```python
from build123d import *

# Parameters (mm, degrees)
SKETCH_1_W          = 150
SKETCH_1_H          = 25
EXTRUDE_2_DEPTH     = 10
SKETCH_5_R          = 5.05
CUT_EXTRUDE_4_DEPTH = 77.689308251
FILLET_1_R          = 12.5


with BuildPart() as part:
    # Эскиз1 → Бобышка-Вытянуть2 (new body)
    with BuildSketch(Plane(origin=(0, 0, 0), x_dir=(1, 0, 0), z_dir=(0, 1, 0))):
        Rectangle(SKETCH_1_W, SKETCH_1_H)
    extrude(amount=EXTRUDE_2_DEPTH)

    # Эскиз5 → Вырез-Вытянуть4 (cut, through all)
    with BuildSketch(Plane(origin=(0, 10, 0), x_dir=(1, 0, 0), z_dir=(0, 1, 0))):
        with Locations(Location((-60, 0, 0), (0, 0, 270))):
            Circle(SKETCH_5_R)
    cut_extrude_4 = extrude(amount=-CUT_EXTRUDE_4_DEPTH, mode=Mode.SUBTRACT)

    # Зеркальное отражение1: Вырез-Вытянуть4 across plane
    add(cut_extrude_4.mirror(Plane(origin=(0, 0, 0), x_dir=(0, 0, 1), z_dir=(1, 0, 0))), mode=Mode.SUBTRACT)

    # Скругление1
    fillet_1_edges = [part.edges().sort_by_distance(p)[0] for p in [
        (-75, 5, 12.5),
        (-75, 5, -12.5),
        (75, 5, 12.5),
        (75, 5, -12.5),
    ]]
    fillet(fillet_1_edges, radius=FILLET_1_R - 0.0001)  # a hair under: the kernel refuses the full size


solid = part.part
```
Geometry: final body of the model. Coordinates: model frame, mm. Round coordinates to 2 decimals unless told otherwise and drop trailing zeros. Order: outer loops, then holes, each group sorted by start corner. A loop starts at its lowest first (then second) coordinate and runs counter-clockwise, first axis right, second up. Notation, with made-up numbers: (14.25, 42.25) - (20.25, 42.25) arc R13 ccw to (20.25, 60.25) - close; hole circle Ø1 at (-27.5, 3.25). An arc over 180 degrees is marked (long way). Write item = value, one per line. Start each with the question number.
Q1. Pull-direction query (X, two-part tool) for faces 1 (the cylindrical face through (64.48, 5.07, 2.33)), 2 (the cylindrical face through (71.241, 5.07, 8.936)), 3 (the cylindrical face through (-71.436, 5.07, 8.741)); classes: +X half, -X half, draft (parallel to the pull), parting line (faces both ways), or undercut.
Q2. Pin query (flat end, axial travel): pin 1 (3 mm diameter, centred on y = 5, z = 7, fed in from -X) (3 decimals); pin 2 (4 mm diameter, centred on x = 10, z = -9, fed in from -Y). Return the tip coordinate at first contact, or that it passes through.
Q3. Ray query, line 1 (X direction, y = 6, z = 0); line 2 (Z direction, x = 60, y = 3); line 3 (X direction, y = 3.25, z = 1). Return the intervals inside material, ascending. Write a range as from..to.
Q4. Cut plane A-A on x = 60. Return the cut outline in (y, z), and give its area (3 significant figures).
Q5. Cut plane B-B on y = 8.25. Give the number of separate pieces and of enclosed holes in the cut face, and give its area (3 significant figures).
Outcome:
q1.face_1 = undercut
q1.face_2 = +X half
q1.face_3 = -X half
q2.pin_1 = -73.725
q2.pin_2 = 0
q3.line_1 = -75..-65.05, -54.95..54.95, 65.05..75
q3.line_2 = -12.5..-5.05, 5.05..12.5
q3.line_3 = -74.96..-64.95, -55.05..55.05, 64.95..74.96
q4.outline = (0, -12.5) - (10, -12.5) - (10, -5.05) - (0, -5.05) - close; (0, 5.05) - (10, 5.05) - (10, 12.5) - (0, 12.5) - close
q4.area = 149 mm^2
q5.separate_pieces = 1
q5.enclosed_holes = 2
q5.area = 3,460 mm^2
